For this review, take the finished solid that the model builds, in its own axes (mm). A direction names the side the tool comes from. Give positions to 0.01 mm unless a question says otherwise; leave off trailing zeros. Loops run counter-clockwise (first coordinate to the right, second up) from the corner with the lowest first, then second, coordinate; pieces in that order, holes last. Notation, with made-up numbers: (22, 22.5) - (44, 22.5) arc R21 cw to (44, 35.5) - close; hole circle Ø5 at (16.5, -40). An arc over 180 degrees is marked (long way). Answer in a Markdown table with one row per item.
```python
from build123d import *

# Parameters (mm, degrees)
SZKIC1_W                          = 100
SZKIC1_H                          = 80
SZKIC1_R                          = 5
DODANIE_WYCI_GNI_CIE1_DEPTH       = 10
SZKIC2_W                          = 60
SZKIC2_H                          = 40
SZKIC2_W_2                        = 50
SZKIC2_H_2                        = 30
WYCI_GNI_CIE_CIENKA_CIANKA1_DEPTH = 125
SZKIC3_R                          = 5
WYTNIJ_WYCI_GNI_CIE1_DEPTH        = 125


with BuildPart() as part:
    # Szkic1 → Dodanie-wyciągnięcie1 (new body)
    with BuildSketch(Plane(origin=(0, 0, 0), x_dir=(1, 0, 0), z_dir=(0, 1, 0))):
        Rectangle(SZKIC1_W, SZKIC1_H)
        with Locations((-39.918726622, 31.934981298)):
            Circle(SZKIC1_R, mode=Mode.SUBTRACT)
        with Locations((39.918726622, 31.934981298)):
            Circle(SZKIC1_R, mode=Mode.SUBTRACT)
        with Locations((39.918726622, -31.934981298)):
            Circle(SZKIC1_R, mode=Mode.SUBTRACT)
        with Locations((-39.918726622, -31.934981298)):
            Circle(SZKIC1_R, mode=Mode.SUBTRACT)
    extrude(amount=DODANIE_WYCI_GNI_CIE1_DEPTH)

    # Szkic2 → Wyciągnięcie-cienka ścianka1 (add)
    with BuildSketch(Plane(origin=(0, 10, 0), x_dir=(1, 0, 0), z_dir=(0, 1, 0))):
        Rectangle(SZKIC2_W, SZKIC2_H)
        Rectangle(SZKIC2_W_2, SZKIC2_H_2, mode=Mode.SUBTRACT)
    extrude(amount=WYCI_GNI_CIE_CIENKA_CIANKA1_DEPTH)

    # Szkic3 → Wytnij-wyciągnięcie1 (cut)
    with BuildSketch(Plane.ZY.offset(30)):
        with Locations((0, 38.229088524)):
            Circle(SZKIC3_R)
        with Locations((0, 73.280775621)):
            Circle(SZKIC3_R)
        with Locations((0, 109.066529463)):
            Circle(SZKIC3_R)
    extrude(amount=-WYTNIJ_WYCI_GNI_CIE1_DEPTH, mode=Mode.SUBTRACT)


solid = part.part
```
1. Clearance check with flat-ended pins moving along their axes: pin 1 (4 mm diameter, centred on x = 7.5, y = 24, fed in from -Z); pin 2 (12 mm diameter, centred on y = 75, z = 3.5, fed in from -X); pin 3 (13 mm diameter, centred on x = 39.92, z = 31.93, fed in from -Y); pin 4 (4 mm diameter, centred on y = 40, z = 9.5, fed in from +X). State where each tip first meets the part, or that it passes through.
Values:
| item | result |
|---|---|
| pin 1 | stops at z = -20 |
| pin 2 | stops at x = -30 |
| pin 3 | stops at y = 0 |
| pin 4 | stops at x = 30 |
2. We need section C-C, the plane z = 0. Count the separate pieces of the cut face and the enclosed holes in it, and give its area (3 significant figures).
Values:
| item | result |
|---|---|
| separate pieces | 7 |
| enclosed holes | 0 |
| area | 1,950 mm^2 |
3. For faces 5 (the face through (-1, 5, -40)), 6 (the face through (25, 72, 7)), 7 (the face through (27.47, 68.4, -1.08)), 8 (the face through (0, 72, 20)), 9 (the face through (0, 72, -20)), list the 3-axis set-ups (+Z, -Z, +X, -X, +Y, -Y) from which the entire face can be reached by the end or side of a thin tool; tool diameter is ignored.
Values:
| item | result |
|---|---|
| face 5 | -Z, +X, -X, +Y, -Y |
| face 6 | +Y |
| face 7 | +X, -X |
| face 8 | +Z, +X, -X, +Y |
| face 9 | -Z, +X, -X, +Y |
4. We need section D-D, the plane x = -31.5. Give the boundary of the cut face in (y, z), and give its area (3 significant figures).
Values:
| item | result |
|---|---|
| outline | (0, -40) - (10, -40) - (10, 40) - (0, 40) - close |
| area | 800 mm^2 |
5. We need section B-B, the plane z = 18.5. Give the boundary of the cut face in (x, y), and give its area (3 significant figures).
Values:
| item | result |
|---|---|
| outline | (-50, 0) - (50, 0) - (50, 10) - (30, 10) - (30, 135) - (-30, 135) - (-30, 10) - (-50, 10) - close |
| area | 8,500 mm^2 |
6. We need section A-A, the plane y = 46.5. Give the boundary of the cut face in (x, z), and give its area (3 significant figures).
Values:
| item | result |
|---|---|
| outline | (-30, -20) - (30, -20) - (30, 20) - (-30, 20) - close; hole (-25, -15) - (25, -15) - (25, 15) - (-25, 15) - close |
| area | 900 mm^2 |
7. Mouldability with a two-part tool opening along Z and no side actions: class faces 1 (the face through (-27.54, 68.4, -1.08)), 2 (the face through (-1, 5, 40)), 3 (the face through (-30, 72, 5)), 4 (the face through (-25, 72, 7)) as released by +Z, released by -Z, zero draft, split by the parting line, or undercut.
Values:
| item | result |
|---|---|
| face 1 | undercut |
| face 2 | released by +Z |
| face 3 | zero draft |
| face 4 | undercut |
8. Wall thickness on line 1 (Y direction, x = -26.6, z = 0); line 2 (Z direction, x = -8, y = 74.5); line 3 (X direction, y = 118.5, z = 5): over which ranges is each line inside the solid? List them lowest first. Write a range as [from, to].
Values:
| item | result |
|---|---|
| line 1 | y = [0, 33.23], [43.23, 68.28], [78.28, 104.07], [114.07, 135] |
| line 2 | z = [-20, -15], [15, 20] |
| line 3 | x = [-30, -25], [25, 30] |
